The listing builds one solid part. Answer for the finished solid, in the listing's coordinates (mm). Coordinates: 2 decimals unless noted, no trailing zeros. Loops run counter-clockwise (first coordinate to the right, second up) from the corner with the lowest first, then second, coordinate; pieces in that order, holes last. Notation, with made-up numbers: M 79.5,51.25 L 124.5,51.25 A21 ccw 124.5,76.25 Z; hole C 34.5,66 d1. An arc over 180 degrees is marked long. Answer in a Markdown table with one row per item. Add a question column.
from build123d import *

# Parameters (mm, degrees)
BOSS_EXTRUDE1_DEPTH   = 3.175
BOSS_EXTRUDE2_DEPTH   = 3.175
F_4_CLEARANCE_HOLE1_D = 2.9464


with BuildPart() as part:
    # Sketch1 → Boss-Extrude1 (new body)
    with BuildSketch(Plane(origin=(0, 0, -14.15699402), x_dir=(-1, 0, 0), z_dir=(0, 0, -1))):
        with BuildLine():
            Line((-49.172312317, -34.502108483), (-53.141062317, -27.628031841))
            ThreePointArc((-53.141062317, -27.628031841), (-55.063803638, -24.012221257), (-56.72992661, -20.271224785))
            ThreePointArc((-56.72992661, -20.271224785), (-54.976138042, -16.13776671), (-50.842679967, -17.891555277))
            ThreePointArc((-50.842679967, -17.891555277), (-49.356678398, -21.228119699), (-47.641801003, -24.453031841))
            Line((-47.641801003, -24.453031841), (-43.673051003, -31.327108483))
            ThreePointArc((-43.673051003, -31.327108483), (-16.68272836, -52.037511462), (17.046778195, -47.596937682))
            Line((17.046778195, -47.596937682), (23.920854837, -43.628187682))
            Line((23.920854837, -43.628187682), (30.79493148, -39.659437682))
            ThreePointArc((30.79493148, -39.659437682), (51.505334458, -12.669115038), (47.064760678, 21.060391517))
            Line((47.064760678, 21.060391517), (43.096010678, 27.934468159))
            ThreePointArc((43.096010678, 27.934468159), (41.160593535, 31.032051618), (39.01404477, 33.987248938))
            ThreePointArc((39.01404477, 33.987248938), (39.561948355, 38.44382292), (44.018522337, 37.895919335))
            ThreePointArc((44.018522337, 37.895919335), (46.425258832, 34.58251628), (48.595271992, 31.109468159))
            Line((48.595271992, 31.109468159), (52.564021992, 24.235391517))
            ThreePointArc((52.564021992, 24.235391517), (57.638963455, -14.312615975), (33.96993148, -45.158698996))
            Line((33.96993148, -45.158698996), (27.095854837, -49.127448996))
            Line((27.095854837, -49.127448996), (20.221778195, -53.096198996))
            ThreePointArc((20.221778195, -53.096198996), (-18.326229296, -58.171140459), (-49.172312317, -34.502108483))
        make_face()
    extrude(amount=BOSS_EXTRUDE1_DEPTH)

    # Sketch6 → Boss-Extrude2 (add)
    with BuildSketch(Plane.XY.offset(-14.15699402)):
        Polygon((67.637194266, -68.918706291), (41.629116859, -87.129758146), (18.471608801, -54.057409171), (44.479686207, -35.846357317), align=None)
        with BuildLine():
            Line((53.079900319, -56.321192451), (55.367208432, -59.587806973))
            ThreePointArc((55.367208432, -59.587806973), (52.622655438, -75.152940473), (37.057521938, -72.408387479))
            Line((37.057521938, -72.408387479), (34.770213825, -69.141772956))
            ThreePointArc((34.770213825, -69.141772956), (37.51476682, -53.576639457), (53.079900319, -56.321192451))
        make_face(mode=Mode.SUBTRACT)
        with BuildLine():
            Line((42.200754795, -82.853533634), (39.913446682, -79.586919112))
            ThreePointArc((39.913446682, -79.586919112), (40.268991048, -77.570526818), (42.285383342, -77.926071183))
            Line((42.285383342, -77.926071183), (44.572691455, -81.192685705))
            ThreePointArc((44.572691455, -81.192685705), (44.21714709, -83.209078), (42.200754795, -82.853533634))
        make_face(mode=Mode.SUBTRACT)
        with BuildLine():
            Line((29.086012958, -59.075416679), (31.373321071, -62.342031201))
            ThreePointArc((31.373321071, -62.342031201), (31.017776706, -64.358423496), (29.001384411, -64.00287913))
            Line((29.001384411, -64.00287913), (26.714076299, -60.736264608))
            ThreePointArc((26.714076299, -60.736264608), (27.069620664, -58.719872314), (29.086012958, -59.075416679))
        make_face(mode=Mode.SUBTRACT)
        with BuildLine():
            Line((47.936667462, -45.876046295), (50.223975575, -49.142660817))
            ThreePointArc((50.223975575, -49.142660817), (49.86843121, -51.159053112), (47.852038915, -50.803508747))
            Line((47.852038915, -50.803508747), (45.564730803, -47.536894224))
            ThreePointArc((45.564730803, -47.536894224), (45.920275168, -45.52050193), (47.936667462, -45.876046295))
        make_face(mode=Mode.SUBTRACT)
        with BuildLine():
            Line((61.136037846, -64.726700799), (63.423345959, -67.993315321))
            ThreePointArc((63.423345959, -67.993315321), (63.067801594, -70.009707616), (61.051409299, -69.654163251))
            Line((61.051409299, -69.654163251), (58.764101186, -66.387548728))
            ThreePointArc((58.764101186, -66.387548728), (59.119645552, -64.371156434), (61.136037846, -64.726700799))
        make_face(mode=Mode.SUBTRACT)
    extrude(amount=-BOSS_EXTRUDE2_DEPTH)

    # #4 Clearance Hole1 (through all)
    with Locations(Plane(origin=(0, 0, -17.33199402), x_dir=(-1, 0, 0), z_dir=(0, 0, -1))):
        with Locations((-53.56643166, -20.541270527), (-47.21643166, -31.539793155), (42.670641335, 35.021229473), (49.020641335, 24.022706845)):
            Hole(F_4_CLEARANCE_HOLE1_D / 2)


solid = part.part
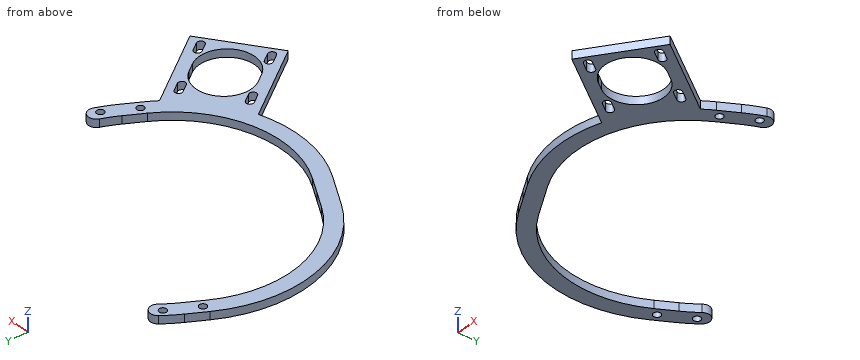
(1) A cutting plane is placed at C-C (y = 0.5). Give the vertices of the cut face in (x, z).
(2) Straight lines are drawn through the part: line 1 (Y direction, x = 42, z = -15); line 2 (X direction, y = -66, z = -17.1); line 3 (X direction, y = -43.5, z = -15.95). For each, find the intervals that lie inside material, in ascending order.
(3) A cutting plane is placed at A-A (x = -15.5). Give the vertices of the cut face in (y, z), plus the area to 3 significant figures.
(4) A cutting plane is placed at B-B (z = -15.7). State how many separate pieces and enclosed holes the cut face has, plus the area to 3 significant figures.
(5) Each of these flat-tipped pins is pushed along its axis until it touches: pin 1 (1.8 mm diameter, centred on x = 53.57, y = -20.54, fed in from +Z) (1 decimal); pin 2 (1 mm diameter, centred on y = -26.5, z = -15, fed in from -X). Where does it stop, or does it pass through?
Solved:
| question | item | result |
|---|---|---|
| 1 | outline | M -59.34,-17.33 L -52.99,-17.33 L -52.99,-14.16 L -59.34,-14.16 Z |
| 2 | line 1 | y = -86.87 to -82.57, -77.62 to -76.35, -51.72 to -34 |
| 2 | line 2 | x = 26.83 to 33.24, 57.39 to 58.57, 62.03 to 65.59 |
| 2 | line 3 | x = -36.65 to -24.14, 33.33 to 49.84 |
| 3 | outline | M -55.5,-17.33 L -48.45,-17.33 L -48.45,-14.16 L -55.5,-14.16 Z |
| 3 | area | 22.4 mm² |
| 4 | separate pieces | 1 |
| 4 | enclosed holes | 9 |
| 4 | area | 1,810 mm² |
| 5 | pin 1 | passes through |
| 5 | pin 2 | stops at x = -52.89 |
